```python
from build123d import *

# Parameters (mm, degrees)
SKETCH1_W           = 60
SKETCH1_H           = 60
BOSS_EXTRUDE1_DEPTH = 100
SKETCH2_R           = 20
BOSS_EXTRUDE2_DEPTH = 50
SKETCH3_W           = 30
SKETCH3_H           = 30
CUT_EXTRUDE1_DEPTH  = 30
SKETCH6_R           = 12.5
CUT_EXTRUDE7_DEPTH  = 40
FILLET1_R           = 10
FILLET2_R           = 10
CHAMFER1_SIZE       = 5
CHAMFER2_SIZE       = 5
CHAMFER2_SIZE2      = 2.886751346


with BuildPart() as part:
    # Sketch1 → Boss-Extrude1 (new body)
    with BuildSketch(Plane(origin=(0, 0, 0), x_dir=(1, 0, 0), z_dir=(0, 1, 0))):
        Rectangle(SKETCH1_W, SKETCH1_H)
    extrude(amount=BOSS_EXTRUDE1_DEPTH)

    # Sketch2 → Boss-Extrude2 (add)
    with BuildSketch(Plane(origin=(0, 100, 0), x_dir=(1, 0, 0), z_dir=(0, 1, 0))):
        with Locations(Location((0, 0, 0), (0, 0, 270))):
            Circle(SKETCH2_R)
    extrude(amount=BOSS_EXTRUDE2_DEPTH)

    # Sketch3 → Cut-Extrude1 (cut)
    with BuildSketch(Plane.XZ):
        with Locations((-0.219000236, 1.191138379)):
            Rectangle(SKETCH3_W, SKETCH3_H)
    extrude(amount=-CUT_EXTRUDE1_DEPTH, mode=Mode.SUBTRACT)

    # Sketch6 → Cut-Extrude7 (cut)
    with BuildSketch(Plane.XZ.offset(-30)):
        with Locations(Location((0, 0, 0), (0, 0, 270))):
            Circle(SKETCH6_R)
    extrude(amount=-CUT_EXTRUDE7_DEPTH, mode=Mode.SUBTRACT)

    # Fillet1
    fillet1_edges = [part.edges().sort_by_distance(p)[0] for p in [
        (-30, 50, -30),
        (-30, 50, 30),
        (30, 50, 30),
        (30, 50, -30),
    ]]
    fillet(fillet1_edges, radius=FILLET1_R)

    # Fillet2
    fillet2_edges = [part.edges().sort_by_distance(p)[0] for p in [
        (-15.219000236, 15, -13.808861621),
        (-15.219000236, 15, 16.191138379),
        (14.780999764, 15, 16.191138379),
        (14.780999764, 15, -13.808861621),
    ]]
    fillet(fillet2_edges, radius=FILLET2_R)

    # Chamfer1
    chamfer1_edges = [part.edges().sort_by_distance(p)[0] for p in [
        (0, 150, -20),
    ]]
    chamfer(chamfer1_edges, length=CHAMFER1_SIZE)

    # Chamfer2
    chamfer2_edges = [part.edges().sort_by_distance(p)[0] for p in [
        (0, 70, 12.5),
    ]]
    chamfer2_side = [part.faces().sort_by_distance(p)[0] for p in [
        (0, 50, 12.5),
    ]]
    chamfer(chamfer2_edges, length=CHAMFER2_SIZE, length2=CHAMFER2_SIZE2, reference=chamfer2_side[0])


solid = part.part
```
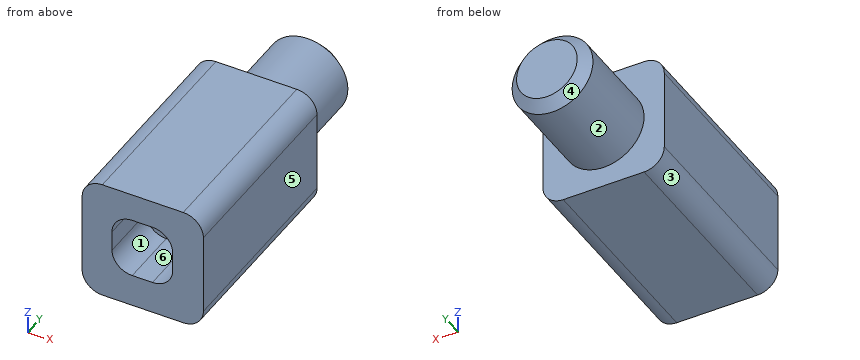
Could you check a few things on this model? Use its own coordinates, in mm. Face numbers are marked on the shaded views. A direction names the side the tool comes from. Round coordinates to 2 decimals unless told otherwise and drop trailing zeros. Write each loop counter-clockwise with the first axis right and the second up, starting at its lowest first coordinate (ties: lowest second). Pieces come first, ordered by that corner, then holes. Notation, with made-up numbers: M 24.5,7 L 59.5,7 A23 cw 59.5,42 Z; hole C 12,6 d1. An arc over 180 degrees is marked long. Answer in a Markdown table with one row per item. Add a question column.
Q1. Will these pins go through, and if not, where does the flat tip stop? pin 1 Ø15 at (x, z) = (-2, 4.5) entering from -Y; pin 2 Ø12 at (y, z) = (100.5, -15) entering from +X; pin 3 Ø2 at (x, y) = (8, 116) entering from -Z (3 decimals); pin 4 Ø1.5 at (x, y) = (-22.5, 92) entering from -Z.
Q2. On a 3-axis mill with a long thin cutter (end or side, diameter ignored), from which of +Z, -Z, +X, -X, +Y, -Y can I reach the whole of each face in a straight line? I mean the marked faces 1, 2 and 3. Say none if no direction works.
Q3. Imagine slicing it at A-A (z = 0). Please give me the cut outline in (x, y), then the cut area to 3 significant figures.
Q4. Imagine slicing it at D-D (y = 79). Please give me the cut outline in (x, z).
Q5. If I drill on line 1 (X direction, y = 38, z = 0); line 2 (X direction, y = 59, z = 8); line 3 (Y direction, x = 16.5, z = 18.5), over which ranges is the centre line in solid material (lowest first)? Write a range as from..to.
Q6. Imagine slicing it at B-B (y = 34.5). Please give me the cut outline in (x, z), then the cut area to 3 significant figures.
Q7. Imagine slicing it at C-C (x = 0). Please give me the cut outline in (y, z).
Q8. If we mould it in two halves opening along X, with no side actions, what happens to the marked faces 4, 5 and 6? For each: +X half, -X half, draft (parallel to the pull), parting line (faces both ways), or undercut.
Values:
| question | item | result |
|---|---|---|
| 1 | pin 1 | y = 65.13 |
| 1 | pin 2 | x = 30 |
| 1 | pin 3 | z = -18.735 |
| 1 | pin 4 | z = -29.85 |
| 2 | face 1 | -Y |
| 2 | face 2 | +Y |
| 2 | face 3 | -Z, -X, +Y, -Y |
| 3 | outline | M -30,0 L -15.22,0 L -15.22,30 L -12.5,30 L -12.5,65 L -9.61,70 L 9.61,70 L 12.5,65 L 12.5,30 L 14.78,30 L 14.78,0 L 30,0 L 30,100 L 20,100 L 20,145 L 15,150 L -15,150 L -20,145 L -20,100 L -30,100 Z |
| 3 | area | 6,090 mm^2 |
| 4 | outline | M -30,-20 A10 ccw -20,-30 L 20,-30 A10 ccw 30,-20 L 30,20 A10 ccw 20,30 L -20,30 A10 ccw -30,20 Z |
| 5 | line 1 | -30..-12.5, 12.5..30 |
| 5 | line 2 | -30..-9.6, 9.6..30 |
| 5 | line 3 | 0..100 |
| 6 | outline | M -30,-20 A10 ccw -20,-30 L 20,-30 A10 ccw 30,-20 L 30,20 A10 ccw 20,30 L -20,30 A10 ccw -30,20 Z; hole C 0,0 d25 |
| 6 | area | 3,020 mm^2 |
| 7 | outline | M 0,-30 L 100,-30 L 100,-20 L 145,-20 L 150,-15 L 150,15 L 145,20 L 100,20 L 100,30 L 0,30 L 0,16.19 L 30,16.19 L 30,12.5 L 65,12.5 L 70,9.61 L 70,-9.61 L 65,-12.5 L 30,-12.5 L 30,-13.81 L 0,-13.81 Z |
| 8 | face 4 | parting line |
| 8 | face 5 | +X half |
| 8 | face 6 | undercut |
